```python
from build123d import *

# Parameters (mm, degrees)
SKETCH1_W           = 41.275
SKETCH1_H           = 1.5875
BOSS_EXTRUDE1_DEPTH = 25.4
SKETCH2_W           = 19.05
SKETCH2_H           = 10.16
CUT_EXTRUDE1_DEPTH  = 25.4


with BuildPart() as part:
    # Sketch1 → Boss-Extrude1 (new body)
    with BuildSketch(Plane(origin=(0, 0, 0), x_dir=(1, 0, 0), z_dir=(0, 1, 0))):
        Polygon((-13.211086677, -8.065885175), (-13.211086677, -6.478385175), (-14.798586677, -6.478385175), (-14.798586677, -23.940885175), (-13.211086677, -23.940885175), align=None)
        with Locations((7.426413323, -7.272135175)):
            Rectangle(SKETCH1_W, SKETCH1_H)
        Polygon((29.651413323, 26.859114825), (28.063913323, 26.859114825), (28.063913323, -6.478385175), (28.063913323, -8.065885175), (29.651413323, -8.065885175), align=None)
    extrude(amount=BOSS_EXTRUDE1_DEPTH)

    # Sketch2 → Cut-Extrude1 (cut)
    with BuildSketch(Plane(origin=(29.651413323, 0, 0), x_dir=(0, 0, -1), z_dir=(1, 0, 0))):
        with Locations((17.334114825, 12.7)):
            Rectangle(SKETCH2_W, SKETCH2_H)
    extrude(amount=-CUT_EXTRUDE1_DEPTH, mode=Mode.SUBTRACT)


solid = part.part
```
The model under review builds one solid part; all positions refer to its coordinate system, in mm. A direction names the side the tool comes from. Give positions to 0.01 mm unless a question says otherwise; leave off trailing zeros. Order: outer loops, then holes, each group sorted by start corner. A loop starts at its lowest first (then second) coordinate and runs counter-clockwise, first axis right, second up. Notation, with made-up numbers: (34.25, 61) - (78.25, 61) arc R14 ccw to (78.25, 81) - close; hole circle Ø4 at (50, 83). An arc over 180 degrees is marked (long way). Use CSV: the item, a comma, the result in double quotes. Start each with the question number.
Q1. We need section D-D, the plane x = -7.5. Write out the cut boundary in (y, z), and give its area (3 significant figures).
Q2. We need section A-A, the plane z = -21.5. Write out the cut boundary in (x, y), and give its area (3 significant figures).
Q3. We need section C-C, the plane z = 17.5. Write out the cut boundary in (x, y), and give its area (3 significant figures).
Q4. Clearance check with flat-ended pins moving along their axes: pin 1 Ø7.5 at (x, y) = (14, 17.5) entering from +Z; pin 2 Ø12.5 at (x, y) = (15, 16) entering from -Z; pin 3 Ø5 at (y, z) = (6, -5) entering from -X. State where each tip first meets the part, or that it passes through.
Q5. The part is to be moulded in two halves that separate along Y. For faces 1 (the flat face through (-14.799, 13, 15)), 2 (the flat face through (29, 17.78, -17)), 3 (the flat face through (10.6, 25.4, 7.8)), say which applies: +Y half, -Y half, draft (parallel to the pull), parting line (faces both ways), or undercut.
Q6. To check wall thickness, follow line 1 along Z through (x, y) = (-0.5, 9.5); line 2 along X through (y, z) = (24, -14); line 3 along X through (y, z) = (7, 21.5). State the ranges of each line that lie inside material, in increasing order. Write a range as [from, to].
Q7. We need section B-B, the plane y = 23. Write out the cut boundary in (x, z).
Q8. Tool access review of faces 4 (the flat face through (8, 13, 8.066)), 5 (the flat face through (-14, 13, 23.941)), 6 (the flat face through (29, 22, -26.859)), 7 (the flat face through (7, 13, 6.478)), 8 (the flat face through (29, 7.62, -17)): name each direction out of +Z, -Z, +X, -X, +Y, -Y from which nothing blocks a thin tool from reaching the whole face with its end or side.
Outcome:
1,outline,"(0, 6.48) - (25.4, 6.48) - (25.4, 8.07) - (0, 8.07) - close"
1,area,"40.3 mm^2"
2,outline,"(28.06, 0) - (29.65, 0) - (29.65, 7.62) - (28.06, 7.62) - close; (28.06, 17.78) - (29.65, 17.78) - (29.65, 25.4) - (28.06, 25.4) - close"
2,area,"24.2 mm^2"
3,outline,"(-14.8, 0) - (-13.21, 0) - (-13.21, 25.4) - (-14.8, 25.4) - close"
3,area,"40.3 mm^2"
4,pin 1,"stops at z = 8.07"
4,pin 2,"stops at z = 6.48"
4,pin 3,"stops at x = 28.06"
5,face 1,"draft"
5,face 2,"undercut"
5,face 3,"+Y half"
6,line 1,"z = [6.48, 8.07]"
6,line 2,"x = [28.06, 29.65]"
6,line 3,"x = [-14.8, -13.21]"
7,outline,"(-14.8, 6.48) - (28.06, 6.48) - (28.06, -26.86) - (29.65, -26.86) - (29.65, 8.07) - (-13.21, 8.07) - (-13.21, 23.94) - (-14.8, 23.94) - close"
8,face 4,"+Z, +X, +Y, -Y"
8,face 5,"+Z, +X, -X, +Y, -Y"
8,face 6,"-Z, +X, -X, +Y, -Y"
8,face 7,"-Z, -X, +Y, -Y"
8,face 8,"-Z, +X, -X"
